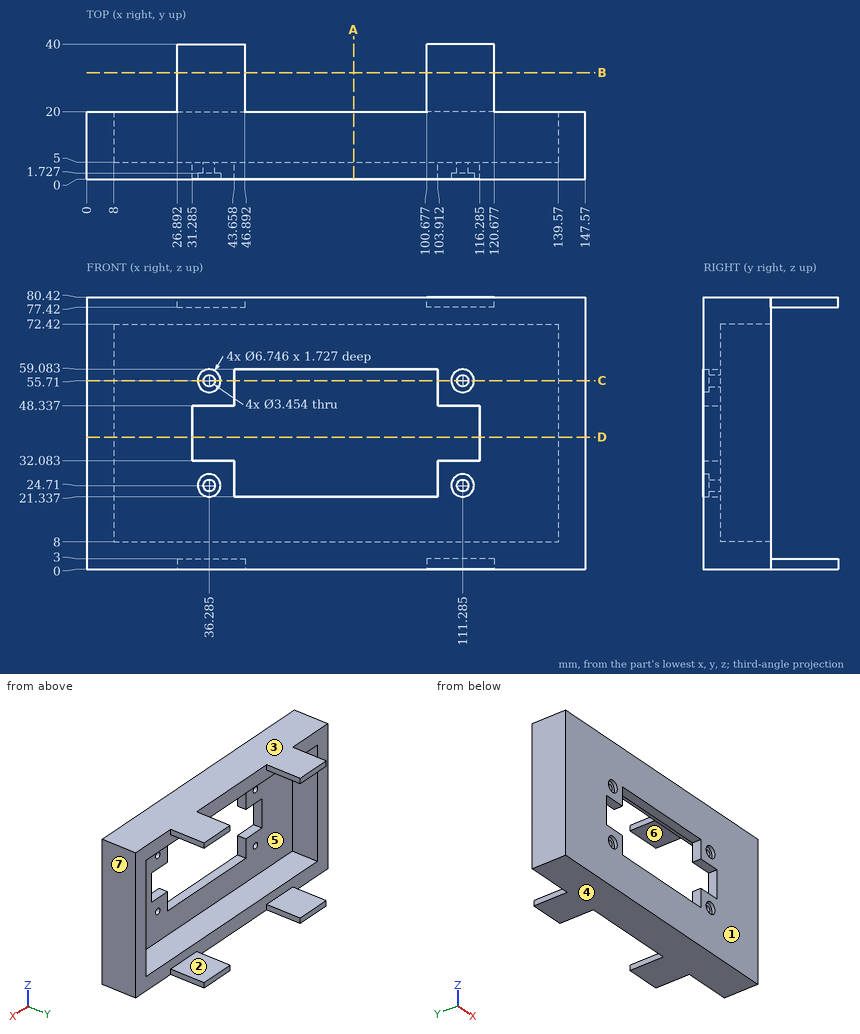
Could you check a few things on this drawing? It's one solid part, dimensions in mm from its lowest x, y, z. A direction names the side the tool comes from. Round coordinates to 2 decimals unless told otherwise and drop trailing zeros. Write each loop counter-clockwise with the first axis right and the second up, starting at its lowest first coordinate (ties: lowest second). Pieces come first, ordered by that corner, then holes. Notation, with made-up numbers: (38.25, -17) -> (78.25, -17) arc R19 ccw to (78.25, 14) -> close; hole circle Ø1 at (65, 13). An arc over 180 degrees is marked (long way). One line per item, written item: value.
1) Suppose I cut it at B-B on y = 31.5. List the corners of the cut face in (x, z) for me, plus the area to 3 significant figures.
Filled sheet:
outline: (26.89, 0) -> (46.89, 0) -> (46.89, 3) -> (26.89, 3) -> close; (26.89, 77.42) -> (46.89, 77.42) -> (46.89, 80.42) -> (26.89, 80.42) -> close; (100.68, 0) -> (120.68, 0) -> (120.68, 3) -> (100.68, 3) -> close; (100.68, 77.42) -> (120.68, 77.42) -> (120.68, 80.42) -> (100.68, 80.42) -> close
area: 240 mm2
2) If I drill on line 1 (X direction, y = 3.2, z = 55.71); line 2 (X direction, y = 12.5, z = 38.5); line 3 (Z direction, x = 84, y = 11), over which ranges is the centre line in solid material (lowest first)? Write a range as [from, to].
Filled sheet:
line 1: x = [0, 34.56], [38.01, 43.66], [103.91, 109.56], [113.01, 147.57]
line 2: x = [0, 8], [139.57, 147.57]
line 3: z = [0, 8], [72.42, 80.42]
3) Suppose I cut it at D-D on z = 39. List the corners of the cut face in (x, y) for me (1 decimal), plus the area to 3 significant figures.
Filled sheet:
outline: (0, 0) -> (31.3, 0) -> (31.3, 5) -> (8, 5) -> (8, 20) -> (0, 20) -> close; (116.3, 0) -> (147.6, 0) -> (147.6, 20) -> (139.6, 20) -> (139.6, 5) -> (116.3, 5) -> close
area: 553 mm2
4) Suppose I cut it at A-A on x = 79. List the corners of the cut face in (y, z) for me.
Filled sheet:
outline: (0, 0) -> (20, 0) -> (20, 8) -> (5, 8) -> (5, 21.34) -> (0, 21.34) -> close; (0, 59.08) -> (5, 59.08) -> (5, 72.42) -> (20, 72.42) -> (20, 80.42) -> (0, 80.42) -> close
5) For the marked faces 5, 6 and 7, which set-ups out of +Z, -Z, +X, -X, +Y, -Y let a thin tool reach every point of the face, with its end or its side?
Filled sheet:
face 5: +Y
face 6: +X, -X, +Y
face 7: +Z, -Z, +X, +Y, -Y
6) We'd pull the mould along Z, two halves only. Please class the marked faces 1, 2, 3 and 4: released by +Z, released by -Z, zero draft, split by the parting line, or undercut.
Filled sheet:
face 1: zero draft
face 2: undercut
face 3: released by +Z
face 4: released by -Z
7) Suppose I cut it at C-C on z = 55.71. List the corners of the cut face in (x, y) for me.
Filled sheet:
outline: (0, 0) -> (32.91, 0) -> (32.91, 1.73) -> (34.56, 1.73) -> (34.56, 5) -> (8, 5) -> (8, 20) -> (0, 20) -> close; (38.01, 1.73) -> (39.66, 1.73) -> (39.66, 0) -> (43.66, 0) -> (43.66, 5) -> (38.01, 5) -> close; (103.91, 0) -> (107.91, 0) -> (107.91, 1.73) -> (109.56, 1.73) -> (109.56, 5) -> (103.91, 5) -> close; (113.01, 1.73) -> (114.66, 1.73) -> (114.66, 0) -> (147.57, 0) -> (147.57, 20) -> (139.57, 20) -> (139.57, 5) -> (113.01, 5) -> close
8) I'm going to push flat-ended pins straight in: pin 1 Ø2.5 at (y, z) = (25.5, 1) entering from +X; pin 2 Ø1.5 at (y, z) = (28.5, 1) entering from -X; pin 3 Ø6 at (x, z) = (113.5, 63) entering from +Y. Where does each tip first touch, or does it pass through?
Filled sheet:
pin 1: stops at x = 120.68
pin 2: stops at x = 26.89
pin 3: stops at y = 5
